Design review of the part built by this model. Coordinates are the model's own, in mm. Round coordinates to 2 decimals unless told otherwise and drop trailing zeros. Order: outer loops, then holes, each group sorted by start corner. A loop starts at its lowest first (then second) coordinate and runs counter-clockwise, first axis right, second up.
from build123d import *

# Parameters (mm, degrees)
F0_R     = 7.1
F0_R_2   = 5.1
F0_R_3   = 1.6
F1_DEPTH = 4
F2_DEPTH = 8.2
F0_R_4   = 11.1
F3_DEPTH = 1
F4_SIZE  = 0.5


with BuildPart() as f1:
    # F0 (on Top) → F1 (new body)
    with BuildSketch(Plane.XY):
        Circle(F0_R)
        Circle(F0_R_2, mode=Mode.SUBTRACT)
        Circle(F0_R_2)
        Circle(F0_R_3, mode=Mode.SUBTRACT)
    extrude(amount=F1_DEPTH)

    # F0 (on Top) → F2 (cut)
    with BuildSketch(Plane.XY):
        Circle(F0_R_2)
        Circle(F0_R_3, mode=Mode.SUBTRACT)
    extrude(amount=F2_DEPTH, mode=Mode.SUBTRACT)

    # F0 (on Top) → F3 (join)
    with BuildSketch(Plane.XY):
        Circle(F0_R_4)
        Circle(F0_R, mode=Mode.SUBTRACT)
    extrude(amount=F3_DEPTH)

    # F4
    f4_edges = [f1.edges().sort_by_distance(p)[0] for p in [
        (-11.1, 0, 1),
    ]]
    chamfer(f4_edges, length=F4_SIZE)


solid = f1.part
1) Clearance check with flat-ended pins moving along their axes: P1, Ø1, axis at y = 8.5, z = 0.5, coming from the -X side; P2, Ø1, axis at x = 5, y = 3.5, coming from the -Z side; P3, Ø1.5, axis at y = 5.5, z = 1.5, coming from the -X side; P4, Ø2, axis at x = -8.5, z = 1.5, coming from the -Y side. State where each tip first meets the part, or that it passes through.
Results:
P1: stops at x = -7.69
P2: stops at z = 0
P3: stops at x = -9.45
P4: stops at y = -7.51
2) The part is to be moulded in two halves that separate along Y. For faces 1 (the face through (2.4, -4.5, 2)), 2 (the face through (-0.92, 7.04, 2.48)), 3 (the face through (7, -2, 1)), say which applies: released by +Y, released by -Y, zero draft, split by the parting line, or undercut.
Results:
face 1: undercut
face 2: split by the parting line
face 3: zero draft
3) Take a section at C-C on z = 2.2. Give the boundary of the cut face in (x, y), plus the area to 3 significant figures.
Results:
outline: circle Ø14.2 at (0, 0); hole circle Ø10.2 at (0, 0)
area: 76.7 mm2
4) To check wall thickness, follow line 1 along Y through (x, z) = (0, 1.4); line 2 along Z through (x, y) = (-3.75, -9); line 3 along Y through (x, z) = (1.75, 2.8). State the ranges of each line that lie inside material, in increasing order.
Results:
line 1: y = -7.1 to -5.1, 5.1 to 7.1
line 2: z = 0 to 1
line 3: y = -6.88 to -4.79, 4.79 to 6.88
5) Take a section at A-A on y = 0. Give the boundary of the cut face in (x, z), plus the area to 4 significant figures.
Results:
outline: (-11.1, 0) - (-5.1, 0) - (-5.1, 4) - (-7.1, 4) - (-7.1, 1) - (-10.6, 1) - (-11.1, 0.5) - close; (5.1, 0) - (11.1, 0) - (11.1, 0.5) - (10.6, 1) - (7.1, 1) - (7.1, 4) - (5.1, 4) - close
area: 23.75 mm2
